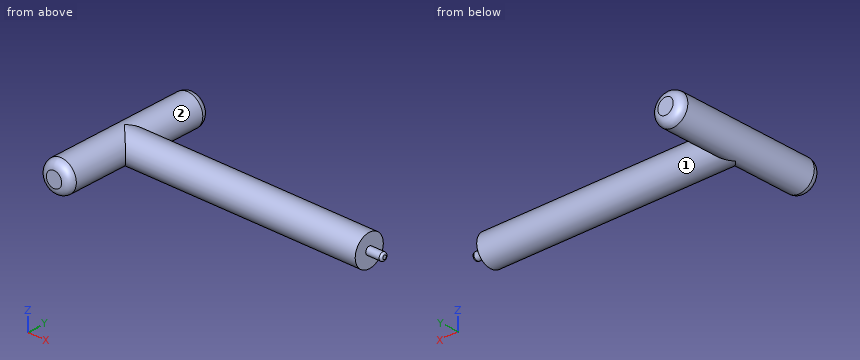
```python
from build123d import *

# Parameters (mm, degrees)
SKETCH1_R                = 12.7
BOSS_EXTRUDE1_DEPTH      = 203.2
SKETCH2_R                = 3.175
BOSS_EXTRUDE2_DEPTH      = 12.7
FILLET2_R                = 1.5875
BOSS_EXTRUDE3_DEPTH      = 63.5
BOSS_EXTRUDE3_DEPTH_BACK = 63.5
SKETCH3_R                = 12.7
FILLET3_R                = 6.35


with BuildPart() as part:
    # Sketch1 → Boss-Extrude1 (new body)
    with BuildSketch(Plane(origin=(0, 0, 0), x_dir=(0, 0, -1), z_dir=(1, 0, 0))):
        Circle(SKETCH1_R)
    extrude(amount=BOSS_EXTRUDE1_DEPTH)

    # Sketch2 → Boss-Extrude2 (add)
    with BuildSketch(Plane(origin=(203.2, 0, 0), x_dir=(0, 0, -1), z_dir=(1, 0, 0))):
        Circle(SKETCH2_R)
    extrude(amount=BOSS_EXTRUDE2_DEPTH)

    # Fillet2
    fillet2_edges = [part.edges().sort_by_distance(p)[0] for p in [
        (215.9, 0, 3.175),
    ]]
    fillet(fillet2_edges, radius=FILLET2_R)

    # Sketch3 → Boss-Extrude3 (add, two sides: drawn at the far end of the back side and taken through both)
    with BuildSketch(Plane(origin=(0, 0, 0), x_dir=(1, 0, 0), z_dir=(0, 1, 0)).offset(-BOSS_EXTRUDE3_DEPTH_BACK)):
        with Locations(Location((0, 0, 0), (0, 0, 270))):
            Circle(SKETCH3_R)
    extrude(amount=BOSS_EXTRUDE3_DEPTH + BOSS_EXTRUDE3_DEPTH_BACK)

    # Fillet3
    # the kernel refuses this fillet: 6.35 mm, written as the material it takes off along each edge
    with BuildSketch(Plane(origin=(0, 63.5, 0), x_dir=(0, 0, 1), z_dir=(-1, 0, 0))) as fillet3_piece_1:
        with BuildLine():
            CenterArc((12.7 - FILLET3_R, -FILLET3_R), FILLET3_R, 0, 90)
            Line((12.7 - FILLET3_R, 0), (12.7, 0))
            Line((12.7, 0), (12.7, -FILLET3_R))
        make_face()
    revolve(axis=Axis((0, 63.5, 0), (0, 1, 0)), mode=Mode.SUBTRACT)
    with BuildSketch(Plane(origin=(0, -63.5, 0), x_dir=(0, 0, 1), z_dir=(-1, 0, 0))) as fillet3_piece_2:
        with BuildLine():
            CenterArc((12.7 - FILLET3_R, FILLET3_R), FILLET3_R, 270, 90)
            Line((12.7 - FILLET3_R, 0), (12.7, 0))
            Line((12.7, 0), (12.7, FILLET3_R))
        make_face()
    revolve(axis=Axis((0, -63.5, 0), (0, 1, 0)), mode=Mode.SUBTRACT)


solid = part.part
```
Build history of the part. All positions in model axes, mm. Face numbers are marked on the shaded views. A direction names the side the tool comes from. Round coordinates to 2 decimals unless told otherwise and drop trailing zeros. Loops run counter-clockwise (first coordinate to the right, second up) from the corner with the lowest first, then second, coordinate; pieces in that order, holes last. Notation, with made-up numbers: M 48,29.5 L 64,29.5 A11 ccw 64,46.5 Z; hole C 15,-37 d5. An arc over 180 degrees is marked long. Answer as CSV lines item,"result".
1. Cut at A-A on y = 43. Write the cut outline in (x, z).
Resolved:
outline,"C 0,0 d25.4"
2. 3-axis set-ups, long thin cutter, end or side, ignore diameter. For the marked faces 1 and 2: which of +Z, -Z, +X, -X, +Y, -Y reach the whole face in a straight line?
Resolved:
face 1,"+X"
face 2,"none"
3. Wall check: probe 1 along Z at (x, y) = (29, 11); probe 2 along X at (y, z) = (-19, 0.75); probe 3 along Y at (x, z) = (2, 6.25). Give the ranges that are in metal, low to high. Write a range as [from, to].
Resolved:
probe 1,"z = [-6.35, 6.35]"
probe 2,"x = [-12.68, 12.68]"
probe 3,"y = [-63.5, 63.5]"
4. Flat gauge pins, fed straight in: P1, Ø12, axis at x = 50, z = 5, coming from the +Y side; P2, Ø2, axis at x = 174, z = -1, coming from the -Y side; P3, Ø4, axis at x = 32, z = 4.5, coming from the +Y side. Where does each tip first touch, or does it go through?
Resolved:
P1,"stops at y = 12.7"
P2,"stops at y = -12.7"
P3,"stops at y = 12.45"
